Geometry check sheet. Reference: the model listing, model coordinates, mm. Face numbers are marked on the shaded views. A direction names the side the tool comes from. Give positions to 0.01 mm unless a question says otherwise; leave off trailing zeros. Loops run counter-clockwise (first coordinate to the right, second up) from the corner with the lowest first, then second, coordinate; pieces in that order, holes last.
Autodesk Inventor part; units mm, degrees
ref_plane "YZ Plane" through (0, 0, 0) normal (1, 0, 0) x (0, 1, 0)
ref_plane "XZ Plane" through (0, 0, 0) normal (0, 1, 0) x (-1, 0, 0)
ref_plane "XY Plane" through (0, 0, 0) normal (0, 0, 1) x (1, 0, 0)
sketch "Szkic1" plane through (0, 0, 0) normal (0, 1, 0) x (-1, 0, 0)
  line L0 (-41, -55) -> (41, -55)
  line L1 (45, -51) -> (45, 51)
  line L2 (41, 55) -> (-41, 55)
  line L3 (-45, 51) -> (-45, -51)
  arc A0 (-41, 55) -> (-45, 51) centre (-41, 51) ccw
  arc A1 (45, 51) -> (41, 55) centre (41, 51) ccw
  arc A2 (41, -55) -> (45, -51) centre (41, -51) ccw
  arc A3 (-45, -51) -> (-41, -55) centre (-41, -51) ccw
  dimension "d14" = 4
  dimension "d15" = 4
  dimension "d16" = 4
  dimension "d17" = 4
extrude "Wyciągnięcie proste1" add sketch "Szkic1" along normal blind 3
sketch "Szkic2" plane through (0, 3, 0) normal (0, 1, 0) x (1, 0, 0)
  circle A0 centre (-30, -36) radius 1.5
  circle A1 centre (-30, -36) radius 3.5
  circle A2 centre (-30, 36) radius 1.5
  circle A3 centre (-30, 36) radius 3.5
  circle A4 centre (30, -36) radius 1.5
  circle A5 centre (30, -36) radius 3.5
  circle A6 centre (30, 36) radius 1.5
  circle A7 centre (30, 36) radius 3.5
  point P0 (0, 0)
  dimension "d24" = 3
  dimension "d25" = 7
extrude "Wyciągnięcie proste2" add sketch "Szkic2" along normal blind 4
sketch "Szkic3" plane through (0, 3, 0) normal (0, 1, 0) x (1, 0, 0)
  circle A0 centre (39, -49) radius 2
  circle A1 centre (-39, -49) radius 2
  circle A2 centre (39, 49) radius 2
  circle A3 centre (-39, 49) radius 2
  point P0 (0, 0)
  dimension "d30" = 4
extrude "Wyciągnięcie proste3" cut sketch "Szkic3" against normal through all
thread "Gwint1"
thread "Gwint2"
thread "Gwint3"
thread "Gwint4"
thread "Gwint5"
thread "Gwint6"
thread "Gwint7"
thread "Gwint8"
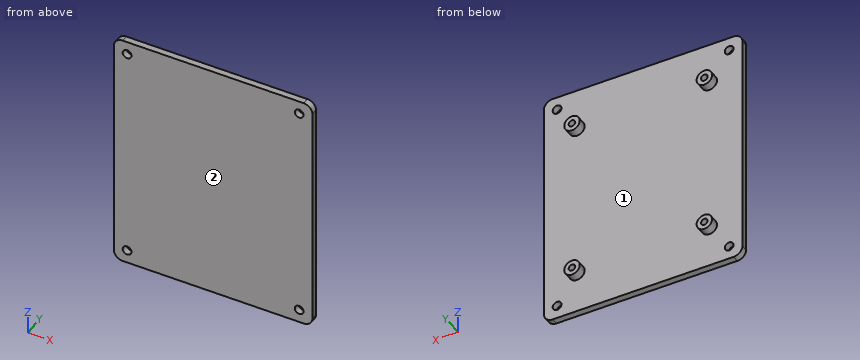
1) Sectioned sample at D-D on z = 36. Enter the section's corners in (x, y), plus the area to 3 significant figures.
2) Sectioned sample at B-B on z = -49. Enter the section's corners in (x, y).
3) Scan lines: line 1 along Z through (x, y) = (-30, 4.7); line 2 along X through (y, z) = (1.5, -49); line 3 along X through (y, z) = (5.7, -36). Record each from-to range of solid material in increasing order.
4) Sectioned sample at A-A on y = 5.5. Enter the section's corners in (x, z), plus the area to 3 significant figures.
5) Depth check by flat-ended pin: P1, Ø3, axis at x = -13.5, z = 16.5, coming from the +Y side; P2, Ø5, axis at x = -30, z = 36, coming from the +Y side. Enter the tip coordinate at first touch or a pass-through.
6) Tool access check on the marked faces 1 and 2. Record the directions out of +Z, -Z, +X, -X, +Y, -Y that give a thin tool (end or side, any length) a straight path to the whole face; none if there is none.
7) Sectioned sample at C-C on x = 30. Enter the section's corners in (y, z).
Determined:
1. outline: (-45, 0) - (45, 0) - (45, 3) - (33.5, 3) - (33.5, 7) - (31.5, 7) - (31.5, 3) - (28.5, 3) - (28.5, 7) - (26.5, 7) - (26.5, 3) - (-26.5, 3) - (-26.5, 7) - (-28.5, 7) - (-28.5, 3) - (-31.5, 3) - (-31.5, 7) - (-33.5, 7) - (-33.5, 3) - (-45, 3) - close
1. area: 302 mm2
2. outline: (-45, 0) - (-41, 0) - (-41, 3) - (-45, 3) - close; (-37, 0) - (37, 0) - (37, 3) - (-37, 3) - close; (41, 0) - (45, 0) - (45, 3) - (41, 3) - close
3. line 1: z = -39.5 to -37.5, -34.5 to -32.5, 32.5 to 34.5, 37.5 to 39.5
3. line 2: x = -45 to -41, -37 to 37, 41 to 45
3. line 3: x = -33.5 to -31.5, -28.5 to -26.5, 26.5 to 28.5, 31.5 to 33.5
4. outline: circle Ø7 at (-30, -36); circle Ø7 at (-30, 36); circle Ø7 at (30, -36); circle Ø7 at (30, 36); hole circle Ø3 at (-30, -36); hole circle Ø3 at (-30, 36); hole circle Ø3 at (30, -36); hole circle Ø3 at (30, 36)
4. area: 126 mm2
5. P1: stops at y = 3
5. P2: stops at y = 7
6. face 1: +Y
6. face 2: +Z, -Z, +X, -X, -Y
7. outline: (0, -55) - (3, -55) - (3, -39.5) - (7, -39.5) - (7, -37.5) - (3, -37.5) - (3, -34.5) - (7, -34.5) - (7, -32.5) - (3, -32.5) - (3, 32.5) - (7, 32.5) - (7, 34.5) - (3, 34.5) - (3, 37.5) - (7, 37.5) - (7, 39.5) - (3, 39.5) - (3, 55) - (0, 55) - close
